Source: CAD feature listing. Evaluate the final solid. Frame: model axes, mm. Coordinates: 2 decimals unless noted, no trailing zeros. Order: outer loops, then holes, each group sorted by start corner. A loop starts at its lowest first (then second) coordinate and runs counter-clockwise, first axis right, second up.
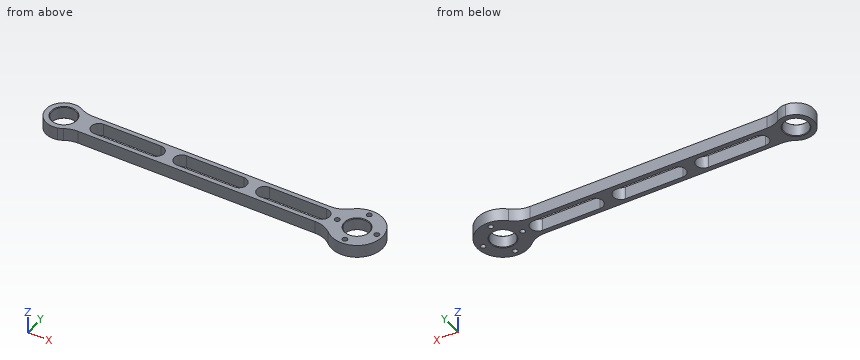
```python
from build123d import *

# Parameters (mm, degrees)
SKETCH_1_R               = 9.5
EXTRUDE_2_DEPTH          = 10
CHAMFER_1_SIZE           = 0.5
CUT_EXTRUDE_1_DEPTH      = 10
SKETCH_3_R               = 2
CUT_EXTRUDE_2_DEPTH      = 10
CHAMFER_2_SIZE           = 0.5
SKETCH_5_R               = 2
CUT_EXTRUDE_3_DEPTH      = 10
CHAMFER_3_SIZE           = 0.5
SKETCH_9_R               = 2
EXTRUDE_3_DEPTH          = 10
SKETCH_10_R              = 2
CUT_EXTRUDE_6_DEPTH      = 10
PATTERN_CIRCULAR_2_COUNT = 4


with BuildPart() as part:
    # Sketch 1 → Extrude 2 (new body)
    with BuildSketch(Plane.XY):
        with BuildLine():
            Line((20.821645942, -9.5), (202.986114682, -9.5))
            ThreePointArc((202.986114682, -9.5), (210.231803055, -10.858648118), (216.493057341, -14.75))
            ThreePointArc((216.493057341, -14.75), (250, 0), (216.493057341, 14.75))
            ThreePointArc((216.493057341, 14.75), (210.231803055, 10.858648118), (202.986114682, 9.5))
            Line((202.986114682, 9.5), (21.63860854, 9.5))
            Line((21.63860854, 9.5), (16.904141504, 9.5))
            ThreePointArc((16.904141504, 9.5), (11.75918395, 10.173090993), (6.960528855, 12.147058824))
            ThreePointArc((6.960528855, 12.147058824), (3.490452231, 13.557903349), (-0.229510749, 13.998118617))
            ThreePointArc((-0.229510749, 13.998118617), (-13.878745314, -1.838594167), (3.423256182, -13.575025492))
            ThreePointArc((3.423256182, -13.575025492), (5.240755683, -12.982083033), (6.960528855, -12.147058824))
            ThreePointArc((6.960528855, -12.147058824), (11.75918395, -10.173090993), (16.904141504, -9.5))
            Line((16.904141504, -9.5), (20.821645942, -9.5))
        make_face()
        Circle(SKETCH_1_R, mode=Mode.SUBTRACT)
        with Locations((230, 0)):
            Circle(SKETCH_1_R, mode=Mode.SUBTRACT)
    extrude(amount=EXTRUDE_2_DEPTH)

    # Chamfer 1
    chamfer_1_edges = [part.edges().sort_by_distance(p)[0] for p in [
        (-9.5, 0, 0),
        (-9.5, 0, 10),
    ]]
    chamfer(chamfer_1_edges, length=CHAMFER_1_SIZE)

    # Sketch 2 → Cut-Extrude 1 (cut)
    with BuildSketch(Plane.XY.offset(10)):
        with BuildLine():
            Line((92.5, -6), (137.5, -6))
            ThreePointArc((137.5, -6), (143.5, 0), (137.5, 6))
            Line((137.5, 6), (92.5, 6))
            ThreePointArc((92.5, 6), (86.5, 0), (92.5, -6))
        make_face()
        with BuildLine():
            Line((157.5, -6), (202.5, -6))
            ThreePointArc((202.5, -6), (208.5, 0), (202.5, 6))
            Line((202.5, 6), (157.5, 6))
            ThreePointArc((157.5, 6), (151.5, 0), (157.5, -6))
        make_face()
        with BuildLine():
            Line((27.5, -6), (72.5, -6))
            ThreePointArc((72.5, -6), (78.5, 0), (72.5, 6))
            Line((72.5, 6), (27.5, 6))
            ThreePointArc((27.5, 6), (21.5, 0), (27.5, -6))
        make_face()
    extrude(amount=-CUT_EXTRUDE_1_DEPTH, mode=Mode.SUBTRACT)

    # Sketch 3 → Cut-Extrude 2 (cut)
    with BuildSketch(Plane.XY.offset(10)):
        with Locations((245, 0)):
            Circle(SKETCH_3_R)
        with Locations((237.5, 12.990381057)):
            Circle(SKETCH_3_R)
        with Locations((222.5, 12.990381057)):
            Circle(SKETCH_3_R)
    extrude(amount=-CUT_EXTRUDE_2_DEPTH, mode=Mode.SUBTRACT)

    # Chamfer 2
    chamfer_2_edges = [part.edges().sort_by_distance(p)[0] for p in [
        (220.5, 0, 10),
    ]]
    chamfer(chamfer_2_edges, length=CHAMFER_2_SIZE)

    # Sketch 5 → Cut-Extrude 3 (cut)
    with BuildSketch(Plane.XY.offset(10)):
        with Locations((215, 0)):
            Circle(SKETCH_5_R)
        with Locations((222.5, -12.990381057)):
            Circle(SKETCH_5_R)
        with Locations((237.5, -12.990381057)):
            Circle(SKETCH_5_R)
    extrude(amount=-CUT_EXTRUDE_3_DEPTH, mode=Mode.SUBTRACT)

    # Chamfer 3
    chamfer_3_edges = [part.edges().sort_by_distance(p)[0] for p in [
        (220.5, 0, 0),
    ]]
    chamfer(chamfer_3_edges, length=CHAMFER_3_SIZE)

    # Sketch 9 → Extrude 3 (add)
    with BuildSketch(Plane.XY.offset(10)):
        with Locations((215, 0)):
            Circle(SKETCH_9_R)
        with Locations((222.5, 12.990381057)):
            Circle(SKETCH_9_R)
        with Locations((237.5, 12.990381057)):
            Circle(SKETCH_9_R)
        with Locations((245, 0)):
            Circle(SKETCH_9_R)
        with Locations((237.5, -12.990381057)):
            Circle(SKETCH_9_R)
        with Locations((222.5, -12.990381057)):
            Circle(SKETCH_9_R)
    extrude(amount=-EXTRUDE_3_DEPTH)

    # Sketch 10 → Cut-Extrude 6 (cut)
    with BuildSketch(Plane.XY.offset(10)):
        with Locations((214.5, 0)):
            Circle(SKETCH_10_R)
    cut_extrude_6 = extrude(amount=-CUT_EXTRUDE_6_DEPTH, mode=Mode.SUBTRACT)

    # Pattern Circular 2: Cut-Extrude 6 ×4 about axis
    pattern_circular_2_axis = Axis((230, 0, 0), (0, 0, 1))
    for i in range(1, PATTERN_CIRCULAR_2_COUNT):
        add(cut_extrude_6.rotate(pattern_circular_2_axis, i * 360 / PATTERN_CIRCULAR_2_COUNT), mode=Mode.SUBTRACT)


solid = part.part
```
Q1. Section query B-B on x = 68. Output: boundary loops of the cut face in (y, z).
Solutions:
outline: (-9.5, 0) - (-6, 0) - (-6, 10) - (-9.5, 10) - close; (6, 0) - (9.5, 0) - (9.5, 10) - (6, 10) - close
Q2. Pin query (flat end, axial travel): P1, Ø8, axis at x = 115, y = 0, coming from the -Z side; P2, Ø3, axis at x = 57.5, z = 4, coming from the -Y side; P3, Ø5, axis at x = 139, z = 5, coming from the +Y side. Return the tip coordinate at first contact, or that it passes through.
Solutions:
P1: passes through
P2: stops at y = -9.5
P3: stops at y = 9.5
Q3. Material intervals for line 1 along Y through (x, z) = (230, 3.75); line 2 along Y through (x, z) = (58.5, 4.25); line 3 along X through (y, z) = (4, 1.5), sorted ascending.
Solutions:
line 1: y = -20 to -17.5, -13.5 to -9.5, 9.5 to 13.5, 17.5 to 20
line 2: y = -9.5 to -6, 6 to 9.5
line 3: x = -13.42 to -8.62, 8.62 to 23.03, 76.97 to 88.03, 141.97 to 153.03, 206.97 to 221.38, 238.62 to 249.6
Q4. Section query A-A on z = 7.5. Give the number of separate pieces and of enclosed holes in the cut face, plus the area to 3 significant figures.
Solutions:
separate pieces: 1
enclosed holes: 9
area: 3,080 mm2
